Study the drawing (mm; zero at the part's minimum x, y, z) and answer. A direction names the side the tool comes from. Round coordinates to 2 decimals unless told otherwise and drop trailing zeros. Loops run counter-clockwise (first coordinate to the right, second up) from the corner with the lowest first, then second, coordinate; pieces in that order, holes last. Notation, with made-up numbers: (79, 49.5) -> (124, 49.5) arc R21 cw to (124, 87.5) -> close; hole circle Ø6 at (42, -31). An arc over 180 degrees is marked (long way). Write each question's results on one line, items separated by ' | '. Start each with the question number.
(1) The part is cut by section C-C (z = 5.5). Determine the outline of the cut face in (x, y).
(2) The part is cut by section D-D (z = 32.5). Determine the outline of the cut face in (x, y).
(3) For the marked faces 1 and 2, determine the directions among +Z, -Z, +X, -X, +Y, -Y from which every point of the face is accessible in a straight line to the end or side of a thin tool.
(4) Straight lines are drawn through the part: probe 1 along X at (y, z) = (4.25, 36); probe 2 along X at (y, z) = (2.5, 2.5); probe 3 along Z at (x, y) = (6.75, 2.75). For each, find the intervals that lie inside material, in ascending order.
(5) A flat-ended cylindrical pin translates along its axis: pin 1 (4 mm diameter, centred on x = 1.5, z = 27.5, fed in from -Y). Find the tip coordinate at first contact, or state that the pin passes through.
(6) The part is cut by section A-A (y = 4). Determine the outline of the cut face in (x, z).
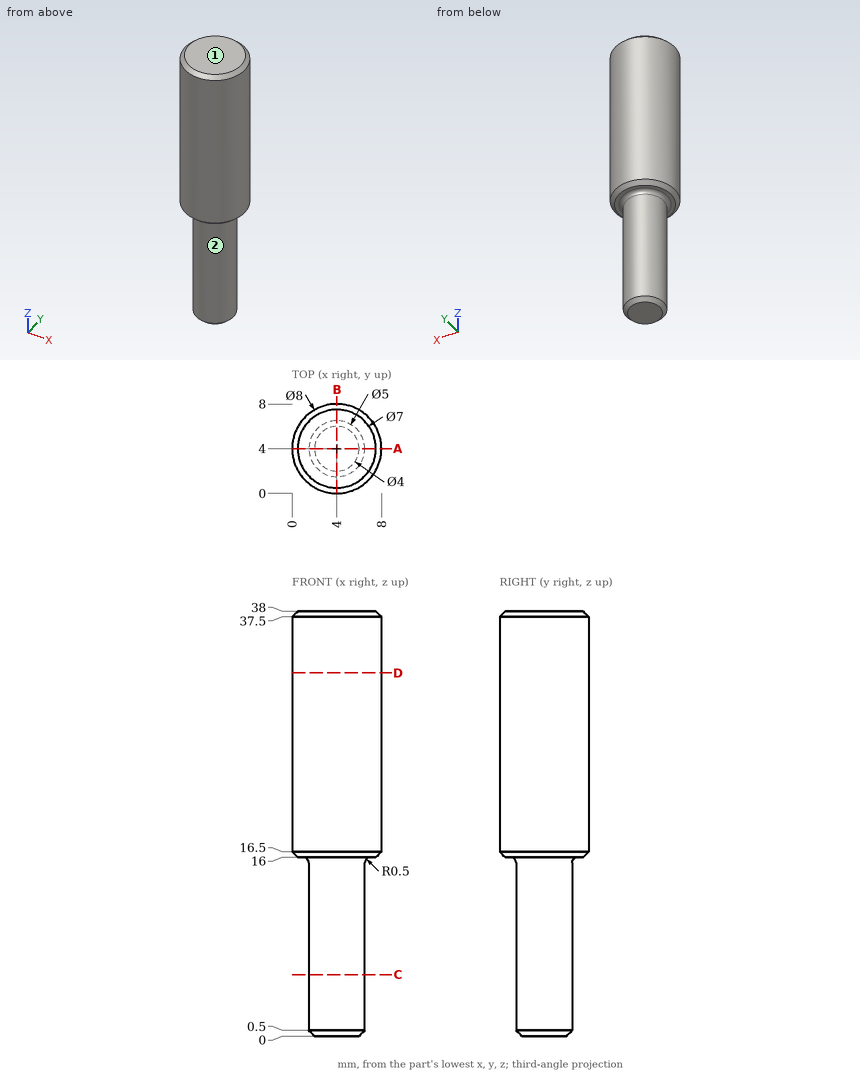
Checked values:
1) outline: circle Ø5 at (4, 4)
2) outline: circle Ø8 at (4, 4)
3) face 1: +Z, +X, -X, +Y, -Y | face 2: -Z
4) probe 1: x = 0.01 to 7.99 | probe 2: x = 2 to 6 | probe 3: z = 16 to 38
5) pin 1: stops at y = 0.03
6) outline: (0, 16.5) -> (0.5, 16) -> (1, 16) arc R0.5 cw to (1.5, 15.5) -> (1.5, 0.5) -> (2, 0) -> (6, 0) -> (6.5, 0.5) -> (6.5, 15.5) arc R0.5 cw to (7, 16) -> (7.5, 16) -> (8, 16.5) -> (8, 37.5) -> (7.5, 38) -> (0.5, 38) -> (0, 37.5) -> close
